from build123d import *

# Parameters (mm, degrees)
BOSS_EXTRUDE1_DEPTH = 130


with BuildPart() as part:
    # Sketch1 → Revolve1 (revolve)
    with BuildSketch(Plane.XY):
        with BuildLine():
            Line((35.74167751, 21.648217086), (31.54167751, 21.648217086))
            ThreePointArc((31.54167751, 21.648217086), (31.095024034, 18.113017357), (29.783135154, 14.8))
            Line((29.783135154, 14.8), (12.463518384, 18))
            Line((12.463518384, 18), (10.54167751, 21.648217086))
            Line((10.54167751, 21.648217086), (-33.810765389, 21.995049121))
            ThreePointArc((-33.810765389, 21.995049121), (-49.094636558, 17.948213618), (-60.198593388, 6.693181934))
            ThreePointArc((-60.198593388, 6.693181934), (-61.144597883, 3.382154176), (-60.497402053, 0))
            Line((-60.497402053, 0), (39.502597947, 0))
            ThreePointArc((39.502597947, 0), (38.55537848, 10.98623941), (35.74167751, 21.648217086))
        make_face()
    revolve(axis=Axis((-90.082052937, 0, 0), (1, 0, 0)))

    # Sketch2 → Boss-Extrude1 (add)
    with BuildSketch(Plane(origin=(0, 0, 0), x_dir=(0, 0, -1), z_dir=(1, 0, 0))):
        Polygon((3.75277675, 0), (1.876388375, 3.25), (-1.876388375, 3.25), (-3.75277675, 0), (-1.876388375, -3.25), (1.876388375, -3.25), align=None)
    extrude(amount=BOSS_EXTRUDE1_DEPTH)


solid = part.part
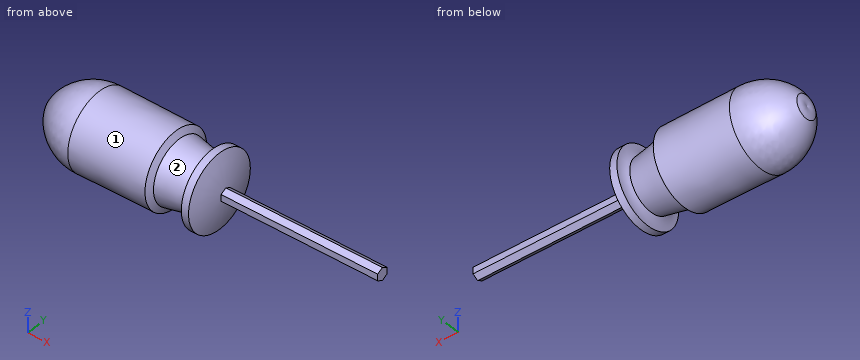
Input: part model. Units: mm. Frame: model coordinates. Face numbers are marked on the shaded views. A direction names the side the tool comes from. Give positions to 0.01 mm unless a question says otherwise; leave off trailing zeros. Loops run counter-clockwise (first coordinate to the right, second up) from the corner with the lowest first, then second, coordinate; pieces in that order, holes last. Notation, with made-up numbers: M 40,87.25 L 73,87.25 A19 ccw 73,101.25 Z; hole C -36,19 d2. An arc over 180 degrees is marked long. Use one line per item in the form item = value.
1. Section query B-B, the plane x = -17.5. Return the cut outline in (y, z) (1 decimal), and give its area (3 significant figures).
Numbers:
outline = C 0,0 d43.7
area = 1,500 mm²
2. First-contact query: pin 1 (3 mm diameter, centred on x = 93.5, z = -0.5, fed in from -Y); pin 2 (3 mm diameter, centred on x = 71, z = -0.5, fed in from +Y); pin 3 (5 mm diameter, centred on x = -30, y = -13.5, fed in from -Z); pin 4 (8 mm diameter, centred on x = 67.5, z = 11.5, fed in from -Y). Flat tips, straight axial feed; report the tip coordinate or a pass-through.
Numbers:
pin_1 = -3.25
pin_2 = 3.25
pin_3 = -19.01
pin_4 = through
3. Section query A-A, the plane x = 108. Return the cut outline in (y, z).
Numbers:
outline = M -3.25,-1.88 L 0,-3.75 L 3.25,-1.88 L 3.25,1.88 L 0,3.75 L -3.25,1.88 Z
4. Line query: L1, parallel to X at y = -3, z = -18.5; L2, parallel to X at y = -6, z = 19; L3, parallel to Z at x = 99, y = 0. Output: solid intervals per line, ascending.
Numbers:
L1 = -47.63 to 12.07, 31.24 to 36.71
L2 = -45 to 11.45, 31.44 to 36.33
L3 = -3.75 to 3.75
5. Reachability of the marked faces 1 and 2 from +Z, -Z, +X, -X, +Y, -Y: full face, straight path, thin tool, end or side. Return the list, or none.
Numbers:
face_1 = +X
face_2 = none
